Verification items for this drawing (mm, ordinates from the low corner). Coordinates: 2 decimals unless noted, no trailing zeros. Loops run counter-clockwise (first coordinate to the right, second up) from the corner with the lowest first, then second, coordinate; pieces in that order, holes last. Notation, with made-up numbers: M 86,48.5 L 125,48.5 A13 ccw 125,54.5 Z; hole C 11.25,41 d4. An arc over 180 degrees is marked long. Write each question's results on one line, items separated by ' | '. Start each with the question number.
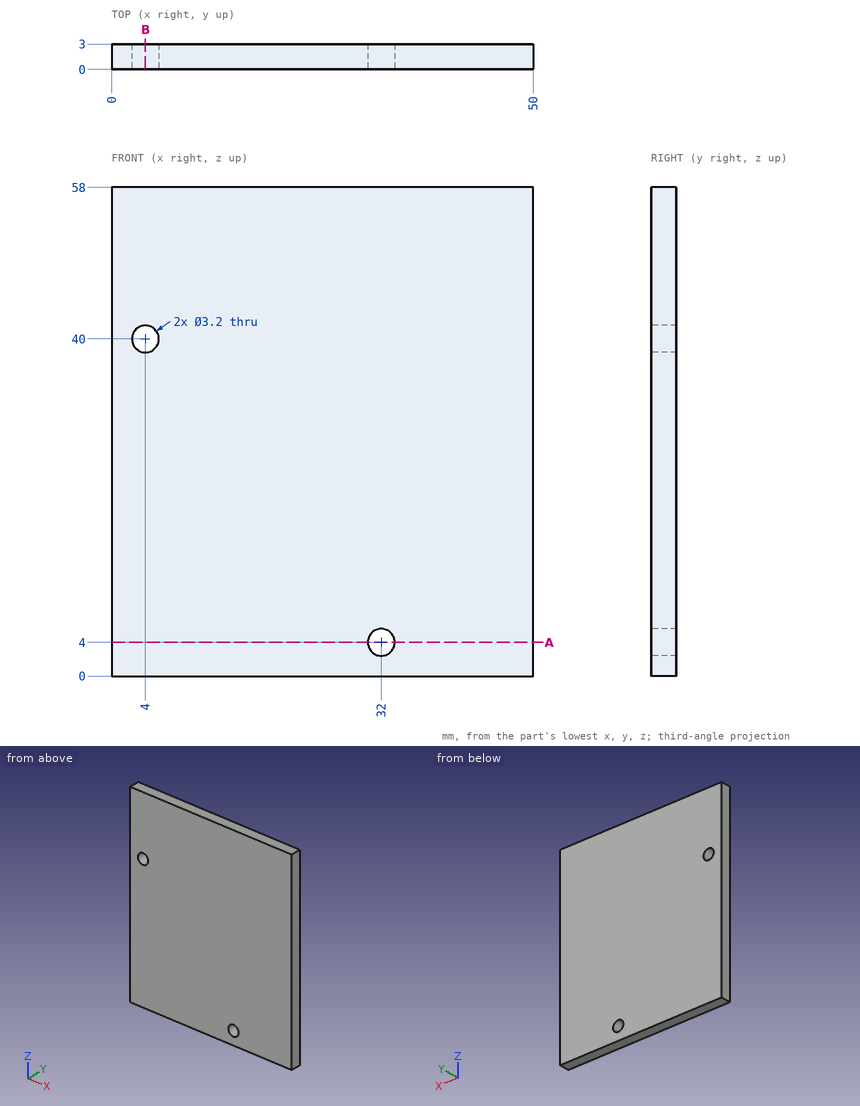
Item 1: Thickness scan on line 1 (X direction, y = 1.65, z = 4); line 2 (X direction, y = 1.4, z = 40). Record the ranges inside material, lowest first.
Item 2: Section check A-A (z = 4). Record the cut outline in (x, y).
Item 3: Section check B-B (x = 4). Record the cut outline in (y, z), plus the area to 3 significant figures.
Computed values:
1) line 1: x = 0 to 30.4, 33.6 to 50 | line 2: x = 0 to 2.4, 5.6 to 50
2) outline: M 0,0 L 30.4,0 L 30.4,3 L 0,3 Z; M 33.6,0 L 50,0 L 50,3 L 33.6,3 Z
3) outline: M 0,0 L 3,0 L 3,38.4 L 0,38.4 Z; M 0,41.6 L 3,41.6 L 3,58 L 0,58 Z | area: 164 mm²
